Autodesk Inventor part; units mm, degrees
ref_plane "Work Plane1" through (63.5, 0, 0) normal (1, 0, 0) x (0, 0, -1)
ref_plane "YZ Plane" through (0, 0, 0) normal (1, 0, 0) x (0, 1, 0)
ref_plane "XZ Plane" through (0, 0, 0) normal (0, 1, 0) x (-1, 0, 0)
sketch "Sketch1" plane through (0, 0, 0) normal (0, 0, 1) x (1, 0, 0)
  line L0 (0, 0) -> (127, 0)
  line L1 (127, 0) -> (127, 127)
  line L2 (127, 127) -> (0, 127)
  line L3 (0, 127) -> (0, 0)
  dimension "d0" = 127
  dimension "d1" = 127
extrude "Extrusion1" add sketch "Sketch1" along normal blind 3.175
sketch "Sketch2" plane through (0, 0, 3.175) normal (0, 0, 1) x (1, 0, 0)
  line L0 (127, 127) -> (0, 127) construction
  line L1 (0, 127) -> (0, 101.6) construction
  line L2 (0, 127) -> (0, 0) construction
  line L3 (0, 0) -> (127, 0) construction
  line L4 (0, 0) -> (0, 25.4) construction
  line L5 (0, 25.4) -> (6.35, 25.4) construction
  line L6 (6.35, 25.4) -> (6.35, 31.75) construction
  line L7 (6.35, 31.75) -> (0, 31.75) construction
  line L8 (0, 31.75) -> (0, 25.4) construction
  line L9 (0, 101.6) -> (6.35, 101.6) construction
  line L10 (6.35, 101.6) -> (6.35, 95.25) construction
  line L11 (6.35, 95.25) -> (0, 95.25) construction
  line L12 (0, 95.25) -> (0, 101.6) construction
  dimension "d4" = 25.4
  dimension "d5" = 25.4
  dimension "d6" = 6.35
  dimension "d7" = 6.35
  dimension "d8" = 6.35
  dimension "d9" = 6.35
ref_plane "Work Plane1" through (63.5, 0, 0) normal (1, 0, 0) x (0, 0, -1)
hole "Hole1" at (6.35, 95.25, 3.175) at (6.35, 31.75, 3.175) direction (0, 0, -1) diameter 3.175 depth 25.4 tip angle 118 countersink diameter 6.35 countersink angle 82
mirror "Mirror1" about plane through (63.5, 0, 0) normal (1, 0, 0) of "Hole1"
properties part number "wheel coreBack"
Verification items for the finished model (mm, model axes). Coordinates: 2 decimals unless noted, no trailing zeros. Order: outer loops, then holes, each group sorted by start corner. A loop starts at its lowest first (then second) coordinate and runs counter-clockwise, first axis right, second up.
Item 1: Material ranges on L1, parallel to X at y = 31.75, z = 0.55; L2, parallel to Y at x = 6.35, z = 0.8, recorded low to high.
Filled in:
L1: x = 0 to 4.76, 7.94 to 119.06, 122.24 to 127
L2: y = 0 to 30.16, 33.34 to 93.66, 96.84 to 127
Item 2: Section check A-A, the plane y = 95.25. Enter the section's corners in (x, z) (1 decimal), then the cut area to 3 significant figures.
Filled in:
outline: (0, 0) - (4.8, 0) - (4.8, 1.3) - (3.2, 3.2) - (0, 3.2) - close; (7.9, 0) - (119.1, 0) - (119.1, 1.3) - (117.5, 3.2) - (9.5, 3.2) - (7.9, 1.3) - close; (122.2, 0) - (127, 0) - (127, 3.2) - (123.8, 3.2) - (122.2, 1.3) - close
area: 377 mm2
Item 3: Release check for a two-part mould opening along X. For faces 1 (the face through (0, 64, 2)), 2 (the face through (7, 30.3, 0.7)), 3 (the face through (64, 127, 2)) record: +X half, -X half, draft (parallel to the pull), parting line (faces both ways), or undercut.
Filled in:
face 1: -X half
face 2: undercut
face 3: draft
Item 4: Depth check by flat-ended pin: pin 1 (4 mm diameter, centred on x = 6.35, y = 95.25, fed in from +Z); pin 2 (3.5 mm diameter, centred on x = 6.35, y = 31.75, fed in from +Z); pin 3 (1.9 mm diameter, centred on x = 120.65, y = 95.25, fed in from +Z). Enter the tip coordinate at first touch or a pass-through.
Filled in:
pin 1: stops at z = 1.82
pin 2: stops at z = 1.54
pin 3: passes through
Item 5: Section check B-B, the plane x = 120.65. Enter the section's corners in (y, z) (1 decimal).
Filled in:
outline: (0, 0) - (30.2, 0) - (30.2, 1.3) - (28.6, 3.2) - (0, 3.2) - close; (33.3, 0) - (93.7, 0) - (93.7, 1.3) - (92.1, 3.2) - (34.9, 3.2) - (33.3, 1.3) - close; (96.8, 0) - (127, 0) - (127, 3.2) - (98.4, 3.2) - (96.8, 1.3) - close
